Build history of the part. All positions in model axes, mm. A direction names the side the tool comes from. Round coordinates to 2 decimals unless told otherwise and drop trailing zeros. Loops run counter-clockwise (first coordinate to the right, second up) from the corner with the lowest first, then second, coordinate; pieces in that order, holes last. Notation, with made-up numbers: M -35,-12 L -5,-12 A18 cw -5,-5 Z; hole C -38.75,72 d6. An arc over 180 degrees is marked long. Use one line per item in the form item = value. Start each with the question number.
Autodesk Inventor part; units mm, degrees
ref_plane "YZ Plane" through (0, 0, 0) normal (1, 0, 0) x (0, 1, 0)
ref_plane "XZ Plane" through (0, 0, 0) normal (0, 1, 0) x (-1, 0, 0)
ref_plane "XY Plane" through (0, 0, 0) normal (0, 0, 1) x (1, 0, 0)
sketch "Sketch1" plane through (0, 0, 0) normal (0, 0, 1) x (1, 0, 0)
  line L0 (-750, 51.5995) -> (750, 51.5995)
  line L1 (750, 51.5995) -> (750, 0)
  line L2 (750, 0) -> (-750, 0)
  line L3 (-750, 0) -> (-750, 51.5995)
  point P0 (0, 0)
  point P1 (0, 0)
  dimension "d0" = 1500
  dimension "d1" = 51.5994
extrude "Plate1" add sketch "Sketch1" along normal blind 2
sketch "Sketch2" plane through (750, 2, 0) normal (0, -1, 0) x (1, 0, 0)
  line L0 (-1500, 0) -> (0, 0)
  line L1 (0, 0) -> (0, 20)
  line L2 (0, 20) -> (-1500, 20)
  line L3 (-1500, 20) -> (-1500, 0)
edge flange "Flange1" height 20 angle 90 thickness 2 bend radius 2.75 thickness toward (0, -1, 0) relief round relief width 2 relief depth 1 edges at (0, 0, 2) wall of the first edge with corners at (-750, 2, 0) (750, 2, 0) (750, 2, 20) (-750, 2, 20)
bend "Bend1"
corner "Corner1"
sketch "Sketch5" plane through (0, 0, 0) normal (0, 0, -1) x (-1, 0, 0)
  line L0 (750, 51.5995) -> (-750, 51.5995)
  line L1 (-1, 30) -> (-1, 51.5995)
  line L2 (750, 0) -> (-750, 0)
  line L3 (-1, 30) -> (1, 30)
  line L4 (1, 30) -> (1, 51.5995)
  point P0 (0, 0)
  point P1 (0, 30)
  point P2 (0, 0)
  dimension "d27" = 2
  dimension "d28" = 30
extrude "Extrusion1" cut sketch "Sketch5" against normal through all
pattern_linear "Rectangular Pattern1" count 3 spacing 500 along (1, 0, 0) of "Extrusion1" first direction both ways yes
sketch "Sketch6" plane through (0, 0, 0) normal (0, 0, -1) x (-1, 0, 0)
  line L0 (-750, 51.5995) -> (-750, 4.75)
  circle A0 centre (-750, 51.5995) radius 22.5
  line L1 (-750, 51.5995) -> (750, 51.5995)
  line L2 (-1, 30) -> (-1, 51.5995) construction
  line L3 (-499, 51.5995) -> (-499, 30) construction
  line L4 (-499, 30) -> (-1, 30) construction
  circle A1 centre (-250, 51.5995) radius 22.5
  point P0 (0, 0)
  point P1 (-727.5, 51.5995)
  point P2 (-750, 29.0995)
  point P3 (-250, 30)
  point P4 (-227.5, 51.5995)
  point P5 (-272.5, 51.5995)
  dimension "d24" = 45
extrude "Extrusion2" cut sketch "Sketch6" against normal through all contours L1 A0 L0 | L1 A1 picked at (-748.3311, 36.7875) picked at (-245.5216, 43.6323)
mirror "Mirror1" about plane through (0, 0, 0) normal (1, 0, 0) of "Extrusion2"
sketch "Sketch7" plane through (0, 0, 2) normal (0, 0, 1) x (1, 0, 0)
  arc A0 (-750, 29.0995) -> (-727.5, 51.5995) centre (-750, 51.5995) ccw
  line L0 (-750, 4.75) -> (-750, 29.0995)
  line L1 (-750, 4.75) -> (750, 4.75)
  line L2 (750, 29.0995) -> (750, 4.75)
  arc A1 (727.5, 51.5995) -> (750, 29.0995) centre (750, 51.5995) ccw
  line L3 (501, 51.5995) -> (727.5, 51.5995)
  line L4 (501, 51.5995) -> (501, 30)
  line L5 (501, 30) -> (499, 30)
  line L6 (499, 30) -> (499, 51.5995)
  line L7 (1, 51.5995) -> (227.5, 51.5995)
  line L8 (1, 51.5995) -> (1, 30)
  line L9 (1, 30) -> (-1, 30)
  line L10 (-1, 30) -> (-1, 51.5995)
  line L11 (-499, 51.5995) -> (-272.5, 51.5995)
  line L12 (-499, 51.5995) -> (-499, 30)
  line L13 (-499, 30) -> (-501, 30)
  line L14 (-501, 30) -> (-501, 51.5995)
  line L15 (-727.5, 51.5995) -> (-501, 51.5995)
  line L16 (650, 4.75) -> (650, 51.5995) construction
  line L17 (-750, 4.75) -> (750, 4.75)
  line L18 (646, 24.7106) -> (650, 31.6388)
  line L19 (650, 31.6388) -> (654, 24.7106)
  line L20 (654, 24.7106) -> (646, 24.7106)
  line L21 (650, 31.6388) -> (650, 24.7106) construction
  line L22 (272.5, 51.5995) -> (499, 51.5995)
  arc A2 (227.5, 51.5995) -> (272.5, 51.5995) centre (250, 51.5995) ccw
  line L23 (-227.5, 51.5995) -> (-1, 51.5995)
  arc A3 (-272.5, 51.5995) -> (-227.5, 51.5995) centre (-250, 51.5995) ccw
  point P0 (0, 0)
  point P1 (650, 28.1747)
  dimension "d29" = 100
  dimension "d30" = 8
extrude "Extrusion3" [suppressed]
mirror "Mirror2" [suppressed]
sketch "Sketch8" plane through (0, 0, 2) normal (0, 0, 1) x (1, 0, 0)
  line L0 (494, 46.5995) -> (494, 34.5995) construction
  line L1 (494, 34.5995) -> (294, 34.5995) construction
  line L2 (294, 34.5995) -> (294, 46.5995) construction
  line L3 (294, 46.5995) -> (494, 46.5995) construction
  line L4 (501, 51.5995) -> (727.5, 51.5995)
  line L5 (272.5, 51.5995) -> (499, 51.5995)
  point P0 (0, 0)
  dimension "d35" = 200
  dimension "d36" = 12
  dimension "d39" = 5
  dimension "d40" = 5
mark "Mark1"
equation "\"d1\" = Стрингер_5"
equation "\"d27\" = d18"
equation "\"d2\" = Thickness"
equation "\"d3\" = BendReliefWidth"
equation "\"d4\" = BendReliefDepth"
equation "\"d5\" = MinimumRemnant"
equation "\"d6\" = TransitionRadius"
equation "\"d9\" = BendRadius"
equation "\"d10\" = CornerReliefSize"
equation "\"d11\" = GapSize"
equation "\"d12\" = JacobiRadiusSize"
equation "\"BendReliefWidth\" = Thickness"
equation "\"BendReliefDepth\" = 0.5 * Thickness"
equation "\"CornerReliefSize\" = 4 * Thickness"
equation "\"MinimumRemnant\" = 2 * Thickness"
equation "\"TransitionRadius\" = BendRadius"
equation "\"JacobiRadiusSize\" = BendRadius"
equation "\"GapSize\" = Thickness"
equation "\"d18\" = Thickness"
properties part number "MSC 065 stringer board ###" material "Stainless Steel"
Q1. Saw through at C-C (z = 13.25). Give the cut face in (x, y), and give its area (3 significant figures).
Q2. Wall check: probe 1 along X at (y, z) = (43, 1.75); probe 2 along Z at (x, y) = (215.5, 16.5). Give the ranges that are in metal, low to high.
Q3. Drop flat-ended pins along their axis: P1, Ø1, axis at y = 42.5, z = 1, coming from the -X side; P2, Ø1.6, axis at y = 43.5, z = 1, coming from the +X side; P3, Ø12, axis at y = 19, z = 13.5, coming from the +X side; P4, Ø1.6, axis at y = 35.5, z = 1, coming from the +X side. Give the stop position or say it passes through.
Q4. Saw through at D-D (x = -156). Give the cut face in (y, z), and give its area (3 significant figures).
Q5. Saw through at A-A (y = 39). Give the cut face in (x, z).
Q6. Tool access for faces 1 (the face through (-10, 29, 0)), 2 (the face through (-10, 29, 2)): list every direction of +Z, -Z, +X, -X, +Y, -Y with a clear straight run to the whole face (end or side of a thin tool).
Q7. Saw through at B-B (x = 250). Give the cut face in (y, z), and give its area (3 significant figures).
Filled in:
q1.outline = M -750,0 L 750,0 L 750,2 L -750,2 Z
q1.area = 3,000 mm²
q2.probe_1 = -729.21 to -501, -499 to -270.79, -229.21 to -1, 1 to 229.21, 270.79 to 499, 501 to 729.21
q2.probe_2 = 0 to 2
q3.P1 = -729.65
q3.P2 = 729.33
q3.P3 = through
q3.P4 = 735.15
q4.outline = M 0,4.75 A4.75 ccw 4.75,0 L 51.6,0 L 51.6,2 L 4.75,2 A2.75 cw 2,4.75 L 2,20 L 0,20 Z
q4.area = 136 mm²
q5.outline = M -731.36,0 L -501,0 L -501,2 L -731.36,2 Z; M -499,0 L -268.64,0 L -268.64,2 L -499,2 Z; M -231.36,0 L -1,0 L -1,2 L -231.36,2 Z; M 1,0 L 231.36,0 L 231.36,2 L 1,2 Z; M 268.64,0 L 499,0 L 499,2 L 268.64,2 Z; M 501,0 L 731.36,0 L 731.36,2 L 501,2 Z
q6.face_1 = -Z, +X, -X, +Y, -Y
q6.face_2 = +Z, +X, -X, +Y
q7.outline = M 0,4.75 A4.75 ccw 4.75,0 L 29.1,0 L 29.1,2 L 4.75,2 A2.75 cw 2,4.75 L 2,20 L 0,20 Z
q7.area = 91.0 mm²
